from build123d import *

# Parameters (mm, degrees)
SKETCH1_R           = 30
SKETCH1_R_2         = 16
SKETCH1_R_3         = 2
BOSS_EXTRUDE1_DEPTH = 10


with BuildPart() as part:
    # Sketch1 → Boss-Extrude1 (new body)
    with BuildSketch(Plane.XY):
        Circle(SKETCH1_R)
        Circle(SKETCH1_R_2, mode=Mode.SUBTRACT)
        with Locations((24, 0)):
            Circle(SKETCH1_R_3, mode=Mode.SUBTRACT)
        with Locations((7.416407865, -22.825356391)):
            Circle(SKETCH1_R_3, mode=Mode.SUBTRACT)
        with Locations((-19.416407865, -14.106846055)):
            Circle(SKETCH1_R_3, mode=Mode.SUBTRACT)
        with Locations((-19.416407865, 14.106846055)):
            Circle(SKETCH1_R_3, mode=Mode.SUBTRACT)
        with Locations((7.416407865, 22.825356391)):
            Circle(SKETCH1_R_3, mode=Mode.SUBTRACT)
    extrude(amount=-BOSS_EXTRUDE1_DEPTH)


solid = part.part
The listing builds one solid part. Answer for the finished solid, in the listing's coordinates (mm). Round coordinates to 2 decimals unless told otherwise and drop trailing zeros. Write each loop counter-clockwise with the first axis right and the second up, starting at its lowest first coordinate (ties: lowest second). Pieces come first, ordered by that corner, then holes. Notation, with made-up numbers: (11, 19) - (17, 19) arc R30 ccw to (17, 44) - close; hole circle Ø2 at (-29.5, 4.5). An arc over 180 degrees is marked (long way). Use a Markdown table: item, result. Add a question column.
1. Consider line 1 (Y direction, x = 0, z = -2); line 2 (X direction, y = 14.5, z = -6.5); line 3 (Y direction, x = 3, z = -4.5). Determine where each line is inside the solid, lowest interval first.
2. The part is cut by section D-D (z = -4.25). Write down the section's boundary in (x, y), and give its area (3 significant figures).
3. For a pull along X with two mould halves and no side action, classify faces 1 (the face through (-29.97, 1.32, -4.93)), 2 (the face through (-18.34, -12.42, -4.93)), 3 (the face through (13, -13, 0)) as +X half, -X half, draft (parallel to the pull), parting line (faces both ways), or undercut.
4. Flat-ended cylindrical pins translate along their axes: P1, Ø1, axis at x = -20.5, z = -6.5, coming from the +Y side; P2, Ø2, axis at x = 9, z = -2, coming from the -Y side; P3, Ø2.5, axis at x = -19.42, y = 14.11, coming from the +Z side; P4, Ø1.5, axis at x = 10.5, z = -4, coming from the -Y side. Find the tip coordinate at first contact, or state that the pin passes through.
5. The part is cut by section C-C (y = -8). Write down the section's boundary in (x, z), and give its area (3 significant figures).
6. The part is cut by section B-B (y = 0). Write down the section's boundary in (x, z), and give its area (3 significant figures).
7. The part is cut by section A-A (x = 24). Write down the section's boundary in (y, z), and give its area (3 significant figures).
Reported:
| question | item | result |
|---|---|---|
| 1 | line 1 | -30 to -16, 16 to 30 |
| 1 | line 2 | -26.26 to -21.38, -17.46 to -6.76, 6.76 to 26.26 |
| 1 | line 3 | -29.85 to -15.72, 15.72 to 29.85 |
| 2 | outline | circle Ø60 at (0, 0); hole circle Ø4 at (-19.42, -14.11); hole circle Ø4 at (-19.42, 14.11); hole circle Ø32 at (0, 0); hole circle Ø4 at (7.42, -22.83); hole circle Ø4 at (7.42, 22.83); hole circle Ø4 at (24, 0) |
| 2 | area | 1,960 mm^2 |
| 3 | face 1 | parting line |
| 3 | face 2 | undercut |
| 3 | face 3 | draft |
| 4 | P1 | y = 22.36 |
| 4 | P2 | y = -28.91 |
| 4 | P3 | through |
| 4 | P4 | y = -28.37 |
| 5 | outline | (-28.91, -10) - (-13.86, -10) - (-13.86, 0) - (-28.91, 0) - close; (13.86, -10) - (28.91, -10) - (28.91, 0) - (13.86, 0) - close |
| 5 | area | 301 mm^2 |
| 6 | outline | (-30, -10) - (-16, -10) - (-16, 0) - (-30, 0) - close; (16, -10) - (22, -10) - (22, 0) - (16, 0) - close; (26, -10) - (30, -10) - (30, 0) - (26, 0) - close |
| 6 | area | 240 mm^2 |
| 7 | outline | (-18, -10) - (-2, -10) - (-2, 0) - (-18, 0) - close; (2, -10) - (18, -10) - (18, 0) - (2, 0) - close |
| 7 | area | 320 mm^2 |
